```python
from build123d import *

# Parameters (mm, degrees)
BOSS_EXTRUDE1_DEPTH = 50
CUT_EXTRUDE1_DEPTH  = 13
FILLET1_R           = 0.2
CUT_EXTRUDE2_DEPTH  = 22.9
BOSS_EXTRUDE2_DEPTH = 2
BOSS_EXTRUDE4_START = -50
BOSS_EXTRUDE4_DEPTH = 2


with BuildPart() as part:
    # Sketch1 → Boss-Extrude1 (new body)
    with BuildSketch(Plane.XY):
        with BuildLine():
            Line((-0.226533162, 0), (-22.9, 0))
            Line((-22.9, 0), (-22.9, 2))
            Line((-22.9, 2), (-1.79756025, 2))
            ThreePointArc((-1.79756025, 2), (-1.552823997, 2.063990635), (-1.370731057, 2.239583333))
            ThreePointArc((-1.370731057, 2.239583333), (-0.802551257, 2.977276557), (-0.088888889, 3.575361503))
            ThreePointArc((-0.088888889, 3.575361503), (-0.023616579, 3.647376483), (0, 3.741657387))
            Line((0, 3.741657387), (0, 4))
            Line((0, 4), (2, 4))
            Line((2, 4), (2, 2.355630783))
            ThreePointArc((2, 2.355630783), (1.987179561, 2.285176459), (1.950361882, 2.223754688))
            Line((1.950361882, 2.223754688), (0.149371544, 0.170309763))
            ThreePointArc((0.149371544, 0.170309763), (-0.020190145, 0.044563331), (-0.226533162, 0))
        make_face()
    extrude(amount=-BOSS_EXTRUDE1_DEPTH)

    # Sketch3 → Loft1 section 0
    with BuildSketch(Plane(origin=(0, 2, 0), x_dir=(1, 0, 0), z_dir=(0, 1, 0))):
        with BuildLine():
            Line((2, 50), (-22.9, 50))
            Line((-22.9, 50), (-22.9, 0))
            Line((-22.9, 0), (2, 0))
            Line((2, 0), (2, 2))
            Line((2, 2), (-20.9, 2))
            Line((-20.9, 2), (-20.9, 48))
            Line((-20.9, 48), (2, 48))
            Line((2, 48), (2, 50))
        make_face()
    # Sketch4 → Loft1 section 1
    with BuildSketch(Plane(origin=(0, 12, 0), x_dir=(-1, 0, 0), z_dir=(0, 1, 0))):
        with BuildLine():
            Line((-2, -50), (31.8, -50))
            Line((31.8, -50), (31.8, 0))
            Line((31.8, 0), (-2, 0))
            Line((-2, 0), (-2, -2))
            Line((-2, -2), (29.8, -2))
            Line((29.8, -2), (29.8, -48))
            Line((29.8, -48), (-2, -48))
            Line((-2, -48), (-2, -50))
        make_face()
    loft()

    # Sketch5 → Cut-Extrude1 (cut)
    with BuildSketch(Plane(origin=(0, 0, 0), x_dir=(0, 0, -1), z_dir=(0.7518094115561124, -0.6593804733957871, 0))):
        Polygon((50, 0.226533162), (0, 0.226533162), (-3.433361375, 0.226533162), (-3.433361375, 4.468376884), (51.426542164, 4.468376884), (51.426542164, 0.226533162), align=None)
    extrude(amount=CUT_EXTRUDE1_DEPTH, mode=Mode.SUBTRACT)

    # Fillet1
    # the kernel refuses this fillet: 0.2 mm, written as the material it takes off along each edge
    with BuildSketch(Plane(origin=(2, 2.28035085, -47.811800168), x_dir=(0, 1, 0), z_dir=(0, 0, -1)), Plane(origin=(2, 2.28035085, 0.188199832), x_dir=(0, 1, 0), z_dir=(0, 0, -1))) as fillet1_piece_1:
        with BuildLine():
            CenterArc((FILLET1_R * 0.376399663711, -FILLET1_R), FILLET1_R, 90, 41.252641273)
            Line((-FILLET1_R * 0.282980809685, -FILLET1_R * 0.248190588444), (0, 0))
            Line((0, 0), (FILLET1_R * 0.376399663711, 0))
        make_face()
    extrude(amount=2.376399664, mode=Mode.SUBTRACT)

    # Sketch6 → Cut-Extrude2 (cut)
    with BuildSketch(Plane(origin=(2, 0, 0), x_dir=(0, 0, -1), z_dir=(1, 0, 0))):
        Polygon((2, 4), (2, 12), (48, 12), (48, 4), (48, -3.389982461), (2, -3.389982461), align=None)
    extrude(amount=-CUT_EXTRUDE2_DEPTH, mode=Mode.SUBTRACT)

    # Sketch7 → Boss-Extrude2 (add)
    with BuildSketch(Plane.XY):
        with BuildLine():
            Line((2, 14.28035085), (2, 12))
            Line((2, 12), (-0.226533162, 12))
            ThreePointArc((-0.226533162, 12), (-0.020190145, 12.044563331), (0.149371544, 12.170309763))
            Line((0.149371544, 12.170309763), (2, 14.28035085))
        make_face()
    extrude(amount=-BOSS_EXTRUDE2_DEPTH)

    # Sketch7<2> → Boss-Extrude4 (add)
    with BuildSketch(Plane.XY.offset(BOSS_EXTRUDE4_START)):
        with BuildLine():
            Line((2, 14.28035085), (2, 12))
            Line((2, 12), (-0.226533162, 12))
            ThreePointArc((-0.226533162, 12), (-0.020190145, 12.044563331), (0.149371544, 12.170309763))
            Line((0.149371544, 12.170309763), (2, 14.28035085))
        make_face()
    extrude(amount=BOSS_EXTRUDE4_DEPTH)


solid = part.part
```
The model under review builds one solid part; all positions refer to its coordinate system, in mm. A direction names the side the tool comes from. Round coordinates to 2 decimals unless told otherwise and drop trailing zeros. Write each loop counter-clockwise with the first axis right and the second up, starting at its lowest first coordinate (ties: lowest second). Pieces come first, ordered by that corner, then holes. Notation, with made-up numbers: (85, 1) - (91, 1) arc R24 ccw to (91, 36) - close; hole circle Ø10 at (60.5, -4). An arc over 180 degrees is marked (long way). Use one line per item in the form item = value.
Q1. Insertion check: pin 1 Ø1.6 at (y, z) = (1.5, -21.5) entering from +X; pin 2 Ø0.6 at (y, z) = (0.5, -17) entering from -X; pin 3 Ø2 at (y, z) = (11, -8) entering from +X; pin 4 Ø8 at (x, z) = (-16, -6.5) entering from -Y. Each pin has a flat end and moves straight along its axis. Give the tip position at first contact, or say it passes through.
Answer key:
pin_1 = -20.9
pin_2 = -22.9
pin_3 = -28.02
pin_4 = through
Q2. For line 1 (Z direction, x = -27, y = 9); line 2 (X direction, y = 1.5, z = -19.5); line 3 (X direction, y = 9.75, z = -46), list the stretches that pass through material, from the lowest coordinate up. Write a range as [from, to].
Answer key:
line_1 = [-50, -48], [-2, 0]
line_2 = [-22.9, -20.9]
line_3 = [-29.8, -27.8]
Q3. Consider section A-A (x = -6.5). State the section outline as (y, z) points, and give its area (3 significant figures).
Answer key:
outline = (0, -50) - (12, -50) - (12, -48) - (0, -48) - close; (0, -2) - (12, -2) - (12, 0) - (0, 0) - close
area = 48.0 mm2
Q4. Tool access review of faces 5 (the flat face through (-31, 12, -25)), 6 (the flat face through (-25.41, 7.07, -24.68)), 7 (the flat face through (-22.9, 1, -25)): name each direction out of +Z, -Z, +X, -X, +Y, -Y from which nothing blocks a thin tool from reaching the whole face with its end or side.
Answer key:
face_5 = +Z, -Z, -X, +Y
face_6 = +X, +Y
face_7 = +Z, -Z, -X, -Y
Q5. Consider section D-D (y = 13). State the section outline as (x, z) points, and give its area (3 significant figures).
Answer key:
outline = (0.88, -50) - (2, -50) - (2, -48) - (0.88, -48) - close; (0.88, -2) - (2, -2) - (2, 0) - (0.88, 0) - close
area = 4.49 mm2
Q6. Consider section B-B (y = 8). State the section outline as (x, z) points, and give its area (3 significant figures).
Answer key:
outline = (-28.24, -50) - (2, -50) - (2, -48) - (-26.24, -48) - (-26.24, -2) - (2, -2) - (2, 0) - (-28.24, 0) - close
area = 213 mm2
Q7. Consider section C-C (z = -41). State the section outline as (x, y) points.
Answer key:
outline = (-31.8, 12) - (-22.9, 2) - (-22.9, 0) - (-20.9, 0) - (-20.9, 2) - (-29.8, 12) - close
Q8. Draft analysis for pull direction Z (two halves, no side actions). For faces 1 (the flat face through (-11, 6, -50)), 2 (the flat face through (-27.41, 7.07, -25.35)), 3 (the flat face through (-10, 6, -48)), 4 (the flat face through (-11, 6, 0)), state which applies: +Z half, -Z half, draft (parallel to the pull), parting line (faces both ways), or undercut.
Answer key:
face_1 = -Z half
face_2 = draft
face_3 = undercut
face_4 = +Z half
